Design review of the part built by this model. Coordinates are the model's own, in mm. Face numbers are marked on the shaded views. Give positions to 0.01 mm unless a question says otherwise; leave off trailing zeros. Write each loop counter-clockwise with the first axis right and the second up, starting at its lowest first coordinate (ties: lowest second). Pieces come first, ordered by that corner, then holes. Notation, with made-up numbers: M 22,24 L 65,24 A24 cw 65,49 Z; hole C -20.5,71 d4. An arc over 180 degrees is marked long. Use one line per item in the form item = value. Start each with the question number.
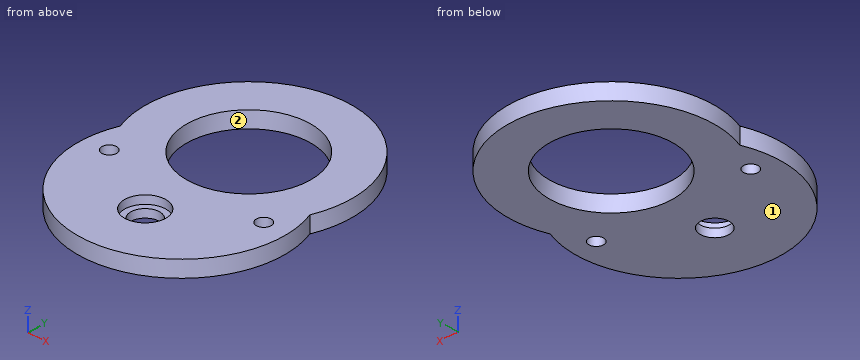
from build123d import *

# Parameters (mm, degrees)
SKETCH_1_R          = 7.5
SKETCH_1_R_2        = 1.75
SKETCH_1_R_3        = 0.9
EXTRUDE_1_DEPTH     = 2
SKETCH_2_R          = 2.5
CUT_EXTRUDE_1_DEPTH = 1


with BuildPart() as part:
    # 草图1 → 凸台-拉伸1 (new body)
    with BuildSketch(Plane.XY):
        with BuildLine():
            ThreePointArc((11.66190379, -4.5), (0, 12.5), (-11.66190379, -4.5))
            ThreePointArc((-11.66190379, -4.5), (0, -21.5), (11.66190379, -4.5))
        make_face()
        Circle(SKETCH_1_R, mode=Mode.SUBTRACT)
        with Locations((0, -13.8)):
            Circle(SKETCH_1_R_2, mode=Mode.SUBTRACT)
        with Locations((-9.5, -8.3)):
            Circle(SKETCH_1_R_3, mode=Mode.SUBTRACT)
        with Locations((9.5, -8.3)):
            Circle(SKETCH_1_R_3, mode=Mode.SUBTRACT)
    extrude(amount=EXTRUDE_1_DEPTH)

    # 草图2 → 切除-拉伸1 (cut)
    with BuildSketch(Plane.XY.offset(2)):
        with Locations((0, -13.8)):
            Circle(SKETCH_2_R)
    extrude(amount=-CUT_EXTRUDE_1_DEPTH, mode=Mode.SUBTRACT)


solid = part.part
1. We need section A-A (y = 0). State the section outline as (x, z) points, and give its area (3 significant figures).
2. To check wall thickness, follow L1, parallel to Y at x = 3.5, z = 1.85; L2, parallel to Y at x = 9.5, z = 1.5; L3, parallel to Z at x = 1.75, y = -13. State the ranges of each line that lie inside material, in increasing order.
3. Draft analysis for pull direction Y (two halves, no side actions). For the marked faces 1 and 2, state which applies: pulls with the +Y half, pulls with the -Y half, needs draft (parallel to the pull), parting line crosses it, or undercut.
4. We need section B-B (x = 0). State the section outline as (y, z) points.
5. We need section D-D (y = -8.3). State the section outline as (x, z) points, and give its area (3 significant figures).
6. We need section C-C (x = -9.5). State the section outline as (y, z) points.
Answer block:
q1.outline = M -12.5,0 L -7.5,0 L -7.5,2 L -12.5,2 Z; M 7.5,0 L 12.5,0 L 12.5,2 L 7.5,2 Z
q1.area = 20.0 mm^2
q2.L1 = -21 to -6.63, 6.63 to 12
q2.L2 = -17.12 to -9.2, -7.4 to 8.12
q2.L3 = 0 to 1
q3.face_1 = needs draft
q3.face_2 = undercut
q4.outline = M -21.5,0 L -15.55,0 L -15.55,1 L -16.3,1 L -16.3,2 L -21.5,2 Z; M -12.05,0 L -7.5,0 L -7.5,2 L -11.3,2 L -11.3,1 L -12.05,1 Z; M 7.5,0 L 12.5,0 L 12.5,2 L 7.5,2 Z
q5.outline = M -12.48,0 L -10.4,0 L -10.4,2 L -12.48,2 Z; M -8.6,0 L 8.6,0 L 8.6,2 L -8.6,2 Z; M 10.4,0 L 12.48,0 L 12.48,2 L 10.4,2 Z
q5.area = 42.7 mm^2
q6.outline = M -17.12,0 L -9.2,0 L -9.2,2 L -17.12,2 Z; M -7.4,0 L 8.12,0 L 8.12,2 L -7.4,2 Z
